from build123d import *

# Parameters (mm, degrees)
EXTRUDE_1_DEPTH     = 1.42
CUT_EXTRUDE_1_REACH = 52.582
SKETCH_2_W          = 32
SKETCH_2_H          = 38.5
SKETCH_2_W_2        = 15.5
SKETCH_2_H_2        = 16.5
CUT_EXTRUDE_2_REACH = 52.582
SKETCH_3_R          = 10
CUT_EXTRUDE_3_REACH = 52.582
CUT_EXTRUDE_4_REACH = 52.582
SKETCH_5_W          = 8
SKETCH_5_H          = 7.5
CUT_EXTRUDE_5_REACH = 52.582
SKETCH_6_W          = 3
SKETCH_6_H          = 5
CUT_EXTRUDE_6_REACH = 52.582
SKETCH_7_W          = 4.5
SKETCH_7_H          = 12


with BuildPart() as part:
    # 草图1 → 凸台-拉伸1 (new body)
    with BuildSketch(Plane.XY):
        with BuildLine():
            Line((-23.82, -42.75), (23.82, -42.75))
            ThreePointArc((23.82, -42.75), (26.068599564, -41.818599564), (27, -39.57))
            Line((27, -39.57), (27, 39.57))
            ThreePointArc((27, 39.57), (26.068599564, 41.818599564), (23.82, 42.75))
            Line((23.82, 42.75), (-23.82, 42.75))
            ThreePointArc((-23.82, 42.75), (-26.068599564, 41.818599564), (-27, 39.57))
            Line((-27, 39.57), (-27, -39.57))
            ThreePointArc((-27, -39.57), (-26.068599564, -41.818599564), (-23.82, -42.75))
        make_face()
    extrude(amount=EXTRUDE_1_DEPTH)

    # 草图2 → 切除-拉伸1 (cut, up to next)
    with BuildSketch(Plane.XY.offset(1.42), mode=Mode.PRIVATE) as cut_extrude_1_sk1:
        with Locations((0, 16)):
            Rectangle(SKETCH_2_W, SKETCH_2_H)
    cut_extrude_1_tool1 = extrude(cut_extrude_1_sk1.sketch, amount=-CUT_EXTRUDE_1_REACH, mode=Mode.PRIVATE) & part.part
    # 草图2 → 切除-拉伸1 (cut, up to next)
    with BuildSketch(Plane.XY.offset(1.42), mode=Mode.PRIVATE) as cut_extrude_1_sk2:
        with Locations((0, -11.5)):
            Rectangle(SKETCH_2_W_2, SKETCH_2_H_2)
    cut_extrude_1_tool2 = extrude(cut_extrude_1_sk2.sketch, amount=-CUT_EXTRUDE_1_REACH, mode=Mode.PRIVATE) & part.part
    add(cut_extrude_1_tool1.solids().sort_by_distance((0, 16, 1.42))[0], mode=Mode.SUBTRACT)
    add(cut_extrude_1_tool2.solids().sort_by_distance((0, -11.5, 1.42))[0], mode=Mode.SUBTRACT)

    # 草图3 → 切除-拉伸2 (cut, up to next)
    with BuildSketch(Plane.XY.offset(1.42), mode=Mode.PRIVATE) as cut_extrude_2_sk1:
        with Locations((-15.95, -27.95)):
            Circle(SKETCH_3_R)
    cut_extrude_2_tool1 = extrude(cut_extrude_2_sk1.sketch, amount=-CUT_EXTRUDE_2_REACH, mode=Mode.PRIVATE) & part.part
    # 草图3 → 切除-拉伸2 (cut, up to next)
    with BuildSketch(Plane.XY.offset(1.42), mode=Mode.PRIVATE) as cut_extrude_2_sk2:
        with BuildLine():
            Line((-18.2, -12.95), (-18.2, -18.206412365))
            ThreePointArc((-18.2, -18.206412365), (-15.95, -17.95), (-13.7, -18.206412365))
            Line((-13.7, -18.206412365), (-13.7, -12.95))
            Line((-13.7, -12.95), (-18.2, -12.95))
        make_face()
    cut_extrude_2_tool2 = extrude(cut_extrude_2_sk2.sketch, amount=-CUT_EXTRUDE_2_REACH, mode=Mode.PRIVATE) & part.part
    add(cut_extrude_2_tool1.solids().sort_by_distance((-15.95, -27.95, 1.42))[0], mode=Mode.SUBTRACT)
    add(cut_extrude_2_tool2.solids().sort_by_distance((-15.95, -15.493086, 1.42))[0], mode=Mode.SUBTRACT)

    # 草图4 → 切除-拉伸3 (cut, up to next)
    with BuildSketch(Plane.XY.offset(1.42), mode=Mode.PRIVATE) as cut_extrude_3_sk1:
        Polygon((-5.45, -20.25), (9.55, -20.25), (9.55, -31.25), (8.05, -31.25), (8.05, -34.75), (-6.05, -34.75), (-6.05, -30.25), (-3.55, -30.25), (-3.55, -27.25), (-5.45, -27.25), align=None)
    cut_extrude_3_tool1 = extrude(cut_extrude_3_sk1.sketch, amount=-CUT_EXTRUDE_3_REACH, mode=Mode.PRIVATE) & part.part
    add(cut_extrude_3_tool1.solids().sort_by_distance((1.958423, -27.392473, 1.42))[0], mode=Mode.SUBTRACT)

    # 草图5 → 切除-拉伸4 (cut, up to next)
    with BuildSketch(Plane.XY.offset(1.42), mode=Mode.PRIVATE) as cut_extrude_4_sk1:
        with Locations((0, -39)):
            Rectangle(SKETCH_5_W, SKETCH_5_H)
    cut_extrude_4_tool1 = extrude(cut_extrude_4_sk1.sketch, amount=-CUT_EXTRUDE_4_REACH, mode=Mode.PRIVATE) & part.part
    add(cut_extrude_4_tool1.solids().sort_by_distance((0, -39, 1.42))[0], mode=Mode.SUBTRACT)

    # 草图6 → 切除-拉伸5 (cut, up to next)
    with BuildSketch(Plane.XY.offset(1.42), mode=Mode.PRIVATE) as cut_extrude_5_sk1:
        with Locations((12, -38.75)):
            Rectangle(SKETCH_6_W, SKETCH_6_H)
    cut_extrude_5_tool1 = extrude(cut_extrude_5_sk1.sketch, amount=-CUT_EXTRUDE_5_REACH, mode=Mode.PRIVATE) & part.part
    # 草图6 → 切除-拉伸5 (cut, up to next)
    with BuildSketch(Plane.XY.offset(1.42), mode=Mode.PRIVATE) as cut_extrude_5_sk2:
        Polygon((17.707106781, -34.767514421), (23.717514421, -28.757106781), (23.717514421, -27.342893219), (17.707106781, -21.332485579), (16.292893219, -21.332485579), (10.282485579, -27.342893219), (10.282485579, -28.757106781), (16.292893219, -34.767514421), align=None)
    cut_extrude_5_tool2 = extrude(cut_extrude_5_sk2.sketch, amount=-CUT_EXTRUDE_5_REACH, mode=Mode.PRIVATE) & part.part
    add(cut_extrude_5_tool1.solids().sort_by_distance((12, -38.75, 1.42))[0], mode=Mode.SUBTRACT)
    add(cut_extrude_5_tool2.solids().sort_by_distance((17, -28.05, 1.42))[0], mode=Mode.SUBTRACT)

    # 草图7 → 切除-拉伸6 (cut, up to next)
    with BuildSketch(Plane.XY.offset(1.42), mode=Mode.PRIVATE) as cut_extrude_6_sk1:
        with Locations((24.75, -18.25)):
            Rectangle(SKETCH_7_W, SKETCH_7_H)
    cut_extrude_6_tool1 = extrude(cut_extrude_6_sk1.sketch, amount=-CUT_EXTRUDE_6_REACH, mode=Mode.PRIVATE) & part.part
    add(cut_extrude_6_tool1.solids().sort_by_distance((24.75, -18.25, 1.42))[0], mode=Mode.SUBTRACT)


solid = part.part
For this review, take the finished solid that the model builds, in its own axes (mm). A direction names the side the tool comes from. Round coordinates to 2 decimals unless told otherwise and drop trailing zeros. Order: outer loops, then holes, each group sorted by start corner. A loop starts at its lowest first (then second) coordinate and runs counter-clockwise, first axis right, second up. Notation, with made-up numbers: M 57.5,57 L 103.5,57 A21 ccw 103.5,95 Z; hole C -23.75,60 d3. An arc over 180 degrees is marked long. Use a Markdown table: item, result. Add a question column.
Item 1: Add section C-C, the plane z = 0.55. State how many separate pieces and enclosed holes the cut face has, then the cut area to 3 significant figures.
Item 2: To check wall thickness, follow line 1 along Y through (x, z) = (-15.95, 0.9); line 2 along Y through (x, z) = (4.5, 1.05); line 3 along X through (y, z) = (-27.95, 1.1). State the ranges of each line that lie inside material, in increasing order.
Item 3: Add section B-B, the plane x = -2.5. Give the boundary of the cut face in (y, z), then the cut area to 3 significant figures.
Item 4: Add section A-A, the plane y = -2. Give the boundary of the cut face in (x, z).
Item 5: Tool access review of faces 5 (the cylindrical face through (26.044, -41.843, 0.7)), 6 (the flat face through (13.33, -24.296, 0.72)): name each direction out of +Z, -Z, +X, -X, +Y, -Y from which nothing blocks a thin tool from reaching the whole face with its end or side.
Item 6: Mouldability with a two-part tool opening along Y and no side actions: class faces 1 (the cylindrical face through (26.093, 41.794, 0.7)), 2 (the flat face through (20.67, -31.804, 0.72)), 3 (the cylindrical face through (-16.36, -37.94, 0.72)), 4 (the flat face through (18, 10, 1.42)) as released by +Y, released by -Y, zero draft, split by the parting line, or undercut.
Geometry results:
| question | item | result |
|---|---|---|
| 1 | separate pieces | 1 |
| 1 | enclosed holes | 5 |
| 1 | area | 2,340 mm² |
| 2 | line 1 | y = -42.75 to -37.95, -12.95 to -3.25, 35.25 to 42.75 |
| 2 | line 2 | y = -42.75 to -34.75, -20.25 to -19.75, 35.25 to 42.75 |
| 2 | line 3 | x = -27 to -25.95, -5.95 to -3.55, 9.55 to 10.28, 23.72 to 27 |
| 3 | outline | M -35.25,0 L -34.75,0 L -34.75,1.42 L -35.25,1.42 Z; M -20.25,0 L -19.75,0 L -19.75,1.42 L -20.25,1.42 Z; M 35.25,0 L 42.75,0 L 42.75,1.42 L 35.25,1.42 Z |
| 3 | area | 12.1 mm² |
| 4 | outline | M -27,0 L -16,0 L -16,1.42 L -27,1.42 Z; M 16,0 L 27,0 L 27,1.42 L 16,1.42 Z |
| 5 | face 5 | +Z, -Z, +X, -Y |
| 5 | face 6 | +Z, -Z |
| 6 | face 1 | released by +Y |
| 6 | face 2 | undercut |
| 6 | face 3 | undercut |
| 6 | face 4 | zero draft |
